Input: part model. Units: mm. Frame: model coordinates. A direction names the side the tool comes from. Give positions to 0.01 mm unless a question says otherwise; leave off trailing zeros. Loops run counter-clockwise (first coordinate to the right, second up) from the corner with the lowest first, then second, coordinate; pieces in that order, holes last. Notation, with made-up numbers: (78.5, 64.5) -> (92.5, 64.5) arc R33 cw to (92.5, 103.5) -> close; hole circle Ø11 at (8, 25). An arc over 180 degrees is marked (long way). Answer as a JSON object with one key per item and string values. Group by question number.
```python
from build123d import *

# Parameters (mm, degrees)
F1_DEPTH = 10
F2_R     = 2.25
F3_DEPTH = 25
F4_R     = 2.25
F5_DEPTH = 3


with BuildPart() as f1:
    # F0 (on Top) → F1 (new body, symmetric)
    with BuildSketch(Plane.XY):
        with BuildLine():
            Line((-35, 7), (-35, 0))
            Line((-35, 0), (-14.456832, 0))
            ThreePointArc((-14.456832, 0), (0, 11), (14.456832, 0))
            Line((14.456832, 0), (35, 0))
            Line((35, 0), (35, 7))
            Line((35, 7), (19.052559, 7))
            ThreePointArc((19.052559, 7), (0, 18), (-19.052559, 7))
            Line((-19.052559, 7), (-35, 7))
        make_face()
    extrude(amount=F1_DEPTH, both=True)

    # F2 (on face) → F3 (cut)
    with BuildSketch(Plane(origin=(0, 7, 0), x_dir=(-1, 0, 0), z_dir=(0, 1, 0))):
        with Locations((-27.026279, 0)):
            Circle(F2_R)
        with Locations((27.026279, 0)):
            Circle(F2_R)
    extrude(amount=-F3_DEPTH, mode=Mode.SUBTRACT)

    # F4 (on face) → F5 (cut)
    with BuildSketch(Plane(origin=(0, 7, 0), x_dir=(-1, 0, 0), z_dir=(0, 1, 0))):
        Polygon((-29.10474, 3.6), (-31.183201, 0), (-29.10474, -3.6), (-24.947818, -3.6), (-22.869358, 0), (-24.947818, 3.6), align=None)
        with Locations((-27.026279, 0)):
            Circle(F4_R, mode=Mode.SUBTRACT)
        Polygon((29.10474, -3.6), (31.183201, 0), (29.10474, 3.6), (24.947818, 3.6), (22.869358, 0), (24.947818, -3.6), align=None)
    extrude(amount=-F5_DEPTH, mode=Mode.SUBTRACT)


solid = f1.part
```
Q1. Ray query, probe 1 along X at (y, z) = (6.75, -0.75); probe 2 along Y at (x, z) = (20, 8.5); probe 3 along Y at (x, z) = (-27.5, 2.75). Return the intervals inside material, ascending.
Q2. Section C-C on z = 1.25. Return the cut outline in (x, y), then the cut area to 3 significant figures.
Q3. Set-up query: faces 5 (the face through (0, 11, 0)), 6 (the face through (31, 7, -2)), 7 (the face through (-23.923, 5.521, 1.825)). Return all of +Z, -Z, +X, -X, +Y, -Y with unobstructed straight access to the full face (end or side cutting, diameter ignored); none if empty.
Q4. Section B-B on z = 6.75. Return the cut outline in (x, y), then the cut area to 3 significant figures.
Q5. Section A-A on y = 9.5. Return the cut outline in (x, z), then the cut area to 3 significant figures.
Q6. Pull-direction query (Z, two-part tool) for faces 1 (the face through (24.88, 2.03, 0.68)), 2 (the face through (-25, 0, 2)), 3 (the face through (-30.16, 5.52, 1.77)), 4 (the face through (0, 13, -10)); classes: +Z half, -Z half, draft (parallel to the pull), parting line (faces both ways), or undercut.
Q7. Section D-D on x = 23.5. Return the cut outline in (y, z).
Q8. Pin query (flat end, axial travel): pin 1 Ø1 at (x, z) = (0, -3.5) entering from -Y; pin 2 Ø1 at (x, y) = (20, 8) entering from -Z; pin 3 Ø6 at (x, z) = (-25.5, -0.5) entering from +Y; pin 4 Ø4 at (y, z) = (15.5, 5) entering from +X. Return the tip coordinate at first contact, or that it passes through.
Numbers:
{
 "1": {"probe 1": "x = -35 to -30.75, -23.3 to -10.46, 10.46 to 23.3, 30.75 to 35", "probe 2": "y = 0 to 7", "probe 3": "y = 0 to 4"},
 "2": {"outline": "(-35, 0) -> (-28.9, 0) -> (-28.9, 4) -> (-30.46, 4) -> (-30.46, 7) -> (-35, 7) -> close; (-25.16, 0) -> (-14.46, 0) arc R15 cw to (14.46, 0) -> (25.16, 0) -> (25.16, 4) -> (23.59, 4) -> (23.59, 7) -> (19.05, 7) arc R22 ccw to (-19.05, 7) -> (-23.59, 7) -> (-23.59, 4) -> (-25.16, 4) -> close; (28.9, 0) -> (35, 0) -> (35, 7) -> (30.46, 7) -> (30.46, 4) -> (28.9, 4) -> close", "area": "481 mm²"},
 "3": {"face 5": "+Z, -Z, -Y", "face 6": "+Z, -Z, +X, +Y", "face 7": "+Y"},
 "4": {"outline": "(-35, 0) -> (-14.46, 0) arc R15 cw to (14.46, 0) -> (35, 0) -> (35, 7) -> (19.05, 7) arc R22 ccw to (-19.05, 7) -> (-35, 7) -> close", "area": "552 mm²"},
 "5": {"outline": "(-17.37, -10) -> (-6.54, -10) -> (-6.54, 10) -> (-17.37, 10) -> close; (6.54, -10) -> (17.37, -10) -> (17.37, 10) -> (6.54, 10) -> close", "area": "433 mm²"},
 "6": {"face 1": "undercut", "face 2": "draft", "face 3": "undercut", "face 4": "-Z half"},
 "7": {"outline": "(0, -10) -> (7, -10) -> (7, -1.09) -> (4, -1.09) -> (4, 1.09) -> (7, 1.09) -> (7, 10) -> (0, 10) -> close"},
 "8": {"pin 1": "stops at y = 10.99", "pin 2": "passes through", "pin 3": "stops at y = 7", "pin 4": "stops at x = 13.33"}
}
